The model under review builds one solid part; all positions refer to its coordinate system, in mm. A direction names the side the tool comes from. Round coordinates to 2 decimals unless told otherwise and drop trailing zeros. Loops run counter-clockwise (first coordinate to the right, second up) from the corner with the lowest first, then second, coordinate; pieces in that order, holes last. Notation, with made-up numbers: (-37.75, -19.75) -> (-23.75, -19.75) arc R21 ccw to (-23.75, 8.25) -> close; hole circle Ø11 at (80, 7.25). An arc over 180 degrees is marked (long way). Use a Markdown table: item, result. Add a question column.
1) For faces 1 (the cylindrical face through (-1.08, -4.88, -0.07)), 2 (the cylindrical face through (10, 3.2, -4.5)), 3 (the flat face through (5, -5, 4)), list the 3-axis set-ups (+Z, -Z, +X, -X, +Y, -Y) from which the entire face can be reached by the end or side of a thin tool; tool diameter is ignored.
2) Wall thickness on probe 1 along Y at (x, z) = (0, 4.6); probe 2 along Y at (x, z) = (0, 2.25); probe 3 along Z at (x, y) = (-6, 5.25): over which ranges is each line inside the solid? List them lowest first.
3) Insertion check: pin 1 (2 mm diameter, centred on x = -2, z = 2.5, fed in from +Y); pin 2 (9 mm diameter, centred on x = 0, y = 0, fed in from -Z); pin 3 (5 mm diameter, centred on y = 9, z = 0.5, fed in from -X). Each pin has a flat end and moves straight along its axis. Give the tip position at first contact, or say it passes through.
4) Mouldability with a two-part tool opening along X and no side actions: class faces 4 (the cylindrical face through (10, 3.2, 4.5)), 5 (the cylindrical face through (11.923, 3.755, 0.07)) as released by +X, released by -X, zero draft, split by the parting line, or undercut.
5) Consider section A-A on y = 0. Give the boundary of the cut face in (x, z), plus the area to 3 significant figures.
6) Consider section D-D on y = -9.5. Give the boundary of the cut face in (x, z).
7) Consider section C-C on z = 0. Give the boundary of the cut face in (x, y), plus the area to 3 significant figures.
from build123d import *

# Parameters (mm, degrees)
SKETCH1_R           = 12.5
SKETCH1_R_2         = 5
BOSS_EXTRUDE1_DEPTH = 5
SKETCH2_R           = 10.5
SKETCH2_R_2         = 6.2
CUT_EXTRUDE1_DEPTH  = 1


with BuildPart() as part:
    # Sketch1 → Boss-Extrude1 (new body, symmetric)
    with BuildSketch(Plane.XY):
        Circle(SKETCH1_R)
        Circle(SKETCH1_R_2, mode=Mode.SUBTRACT)
    extrude(amount=BOSS_EXTRUDE1_DEPTH, both=True)

    # Sketch2 → Cut-Extrude1 (cut)
    with BuildSketch(Plane.XY.offset(5)):
        Circle(SKETCH2_R)
        Circle(SKETCH2_R_2, mode=Mode.SUBTRACT)
    cut_extrude1 = extrude(amount=-CUT_EXTRUDE1_DEPTH, mode=Mode.SUBTRACT)

    # Mirror1: Cut-Extrude1 across plane
    add(cut_extrude1.mirror(Plane.XY), mode=Mode.SUBTRACT)


solid = part.part
Result set:
| question | item | result |
|---|---|---|
| 1 | face 1 | +Z, -Z |
| 1 | face 2 | -Z |
| 1 | face 3 | +Z |
| 2 | probe 1 | -12.5 to -10.5, -6.2 to -5, 5 to 6.2, 10.5 to 12.5 |
| 2 | probe 2 | -12.5 to -5, 5 to 12.5 |
| 2 | probe 3 | -4 to 4 |
| 3 | pin 1 | y = 12.46 |
| 3 | pin 2 | through |
| 3 | pin 3 | x = -10.68 |
| 4 | face 4 | undercut |
| 4 | face 5 | split by the parting line |
| 5 | outline | (-12.5, -5) -> (-10.5, -5) -> (-10.5, -4) -> (-6.2, -4) -> (-6.2, -5) -> (-5, -5) -> (-5, 5) -> (-6.2, 5) -> (-6.2, 4) -> (-10.5, 4) -> (-10.5, 5) -> (-12.5, 5) -> close; (5, -5) -> (6.2, -5) -> (6.2, -4) -> (10.5, -4) -> (10.5, -5) -> (12.5, -5) -> (12.5, 5) -> (10.5, 5) -> (10.5, 4) -> (6.2, 4) -> (6.2, 5) -> (5, 5) -> close |
| 5 | area | 133 mm2 |
| 6 | outline | (-8.12, -5) -> (-4.47, -5) -> (-4.47, -4) -> (4.47, -4) -> (4.47, -5) -> (8.12, -5) -> (8.12, 5) -> (4.47, 5) -> (4.47, 4) -> (-4.47, 4) -> (-4.47, 5) -> (-8.12, 5) -> close |
| 7 | outline | circle Ø25 at (0, 0); hole circle Ø10 at (0, 0) |
| 7 | area | 412 mm2 |
